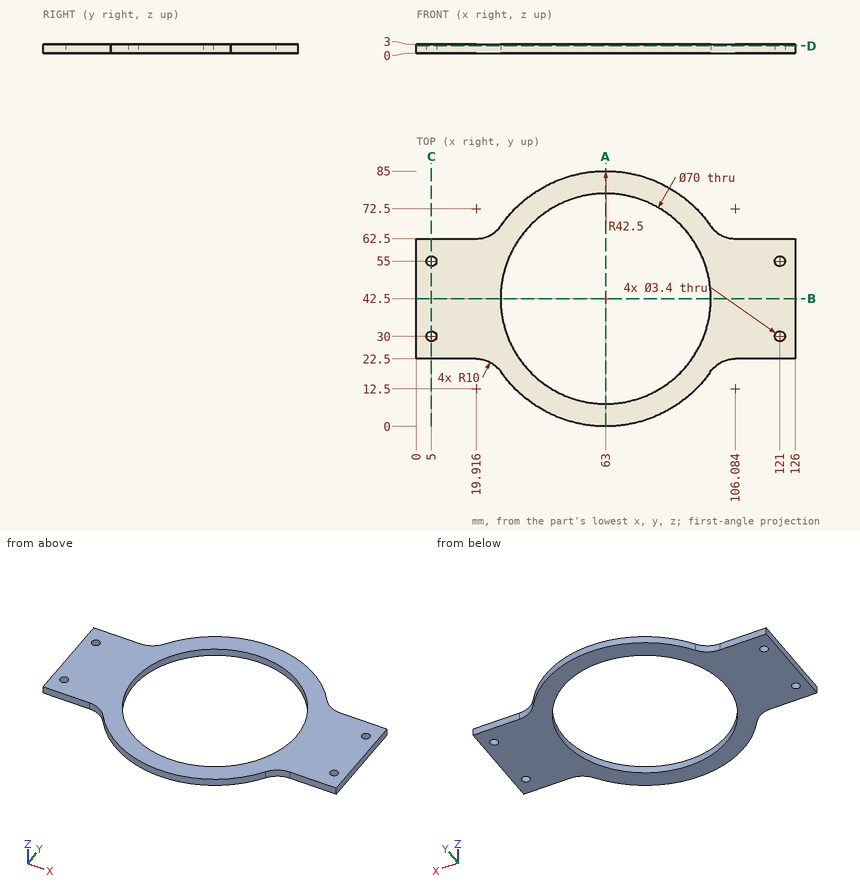
The figure shows three views and two pictorial views of one solid part (mm, origin at its lowest corner). Answer the questions. Give positions to 0.01 mm unless a question says otherwise; leave off trailing zeros. Write each loop counter-clockwise with the first axis right and the second up, starting at its lowest first coordinate (ties: lowest second). Pieces come first, ordered by that corner, then holes. Notation, with made-up numbers: (-22, 45) - (16, 45) arc R14 ccw to (16, 51) - close; hole circle Ø3 at (70, -10.75). An arc over 180 degrees is marked (long way). Use one line per item in the form item = value.
1. Consider L1, parallel to Y at x = 121, z = 0.75; L2, parallel to X at y = 42, z = 1.15; L3, parallel to Y at x = 63, z = 0.65. Determine where each line is inside the solid, lowest interval first.
Filled in:
L1 = 22.5 to 28.3, 31.7 to 53.3, 56.7 to 62.5
L2 = 0 to 28, 98 to 126
L3 = 0 to 7.5, 77.5 to 85
2. A cutting plane is placed at A-A (x = 63). Write down the section's boundary in (y, z).
Filled in:
outline = (0, 0) - (7.5, 0) - (7.5, 3) - (0, 3) - close; (77.5, 0) - (85, 0) - (85, 3) - (77.5, 3) - close
3. A cutting plane is placed at B-B (y = 42.5). Write down the section's boundary in (x, z), and give its area (3 significant figures).
Filled in:
outline = (0, 0) - (28, 0) - (28, 3) - (0, 3) - close; (98, 0) - (126, 0) - (126, 3) - (98, 3) - close
area = 168 mm^2
4. A cutting plane is placed at C-C (x = 5). Write down the section's boundary in (y, z).
Filled in:
outline = (22.5, 0) - (28.3, 0) - (28.3, 3) - (22.5, 3) - close; (31.7, 0) - (53.3, 0) - (53.3, 3) - (31.7, 3) - close; (56.7, 0) - (62.5, 0) - (62.5, 3) - (56.7, 3) - close
5. A cutting plane is placed at D-D (z = 2.4). Write down the section's boundary in (x, y).
Filled in:
outline = (0, 22.5) - (19.92, 22.5) arc R10 cw to (28.12, 18.21) arc R42.5 ccw to (97.88, 18.21) arc R10 cw to (106.08, 22.5) - (126, 22.5) - (126, 62.5) - (106.08, 62.5) arc R10 cw to (97.88, 66.79) arc R42.5 ccw to (28.12, 66.79) arc R10 cw to (19.92, 62.5) - (0, 62.5) - close; hole circle Ø3.4 at (5, 30); hole circle Ø3.4 at (5, 55); hole circle Ø70 at (63, 42.5); hole circle Ø3.4 at (121, 30); hole circle Ø3.4 at (121, 55)
6. Each of these flat-tipped pins is pushed along its axis until it touches: pin 1 Ø1.5 at (x, z) = (9, 1.5) entering from -Y; pin 2 Ø4 at (x, y) = (5, 30) entering from -Z; pin 3 Ø1.5 at (x, z) = (116, 1.5) entering from +Y. Where does it stop, or does it pass through?
Filled in:
pin_1 = 22.5
pin_2 = 0
pin_3 = 62.5
